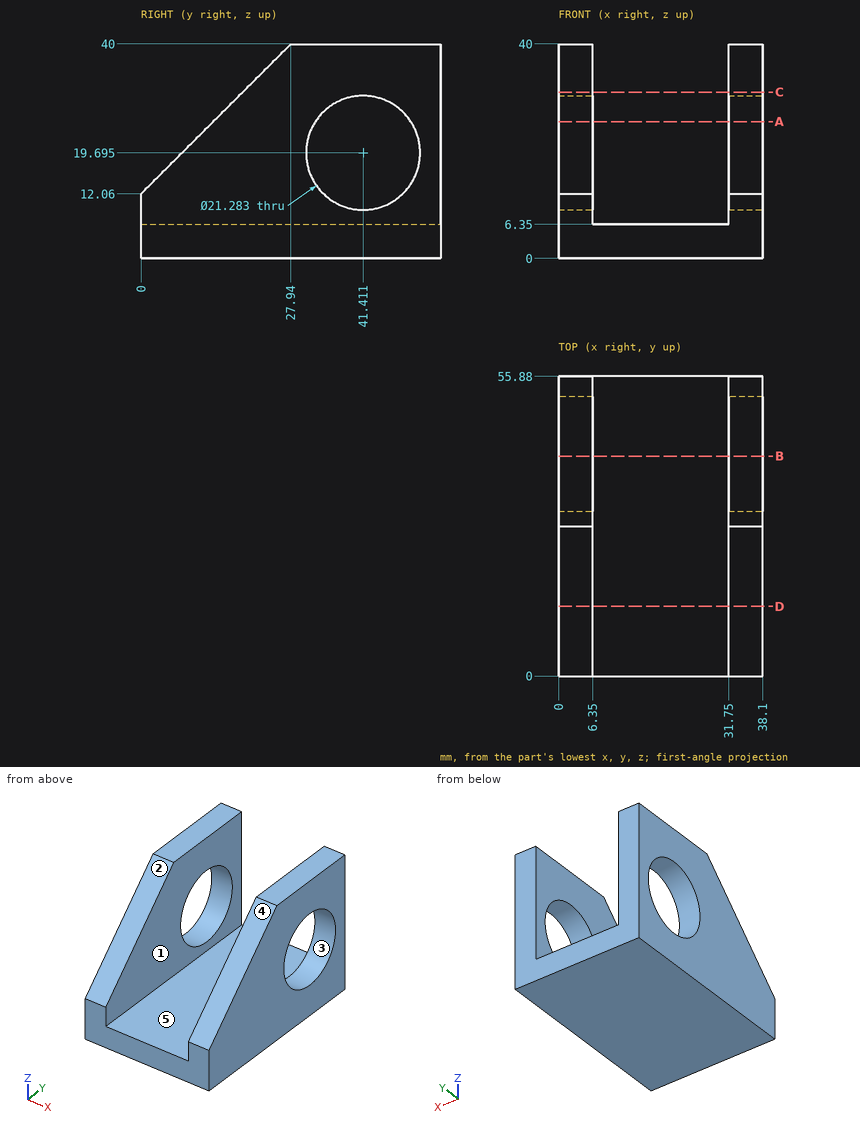
The figure shows three views and two pictorial views of one solid part (mm, origin at its lowest corner). Answer the questions. A direction names the side the tool comes from. Coordinates: 2 decimals unless noted, no trailing zeros. Loops run counter-clockwise (first coordinate to the right, second up) from the corner with the lowest first, then second, coordinate; pieces in that order, holes last. Notation, with made-up numbers: (0.25, 24) -> (19.25, 24) arc R24 ccw to (19.25, 39) -> close; hole circle Ø6 at (3.5, -12.5). An arc over 180 degrees is marked (long way). Write item = value, one per line. Start each with the question number.
1) A cutting plane is placed at C-C (z = 31). Give the vertices of the cut face in (x, y).
2) Given pin 1 Ø13 at (y, z) = (41.41, 19.7) entering from +X; pin 2 Ø3 at (x, y) = (17, 40.5) entering from +Z, each flat-ended and moving along its own axis, determine where each tip first touches the part or whether it passes through.
3) A tool of negligible diameter and unlimited length cuts with its end or side. For the marked faces 4 and 5, from which of +Z, -Z, +X, -X, +Y, -Y can it reach the whole face along a straight path? Write none if from no direction.
4) A cutting plane is placed at D-D (y = 13). Give the vertices of the cut face in (x, z).
5) Straight lines are drawn through the part: line 1 (X direction, y = 47, z = 36.5); line 2 (Z direction, x = 15, y = 22.5); line 3 (Z direction, x = 32, y = 50). For each, find the intervals that lie inside material, in ascending order. Write a range as from..to.
6) A cutting plane is placed at B-B (y = 41). Give the vertices of the cut face in (x, z), then the cut area to 3 significant figures.
7) A cutting plane is placed at A-A (z = 25.5). Give the vertices of the cut face in (x, y).
8) The mould has two halves that part along Y. Classify the marked faces 1, 2 and 3: released by +Y, released by -Y, zero draft, split by the parting line, or undercut.
Responses:
q1.outline = (0, 18.94) -> (6.35, 18.94) -> (6.35, 55.88) -> (0, 55.88) -> close; (31.75, 18.94) -> (38.1, 18.94) -> (38.1, 55.88) -> (31.75, 55.88) -> close
q2.pin_1 = through
q2.pin_2 = 6.35
q3.face_4 = +Z, +X, -X, -Y
q3.face_5 = +Z, +Y, -Y
q4.outline = (0, 0) -> (38.1, 0) -> (38.1, 25.06) -> (31.75, 25.06) -> (31.75, 6.35) -> (6.35, 6.35) -> (6.35, 25.06) -> (0, 25.06) -> close
q5.line_1 = 0..6.35, 31.75..38.1
q5.line_2 = 0..6.35
q5.line_3 = 0..13.41, 25.98..40
q6.outline = (0, 0) -> (38.1, 0) -> (38.1, 9.06) -> (31.75, 9.06) -> (31.75, 6.35) -> (6.35, 6.35) -> (6.35, 9.06) -> (0, 9.06) -> close; (0, 30.33) -> (6.35, 30.33) -> (6.35, 40) -> (0, 40) -> close; (31.75, 30.33) -> (38.1, 30.33) -> (38.1, 40) -> (31.75, 40) -> close
q6.area = 399 mm²
q7.outline = (0, 13.44) -> (6.35, 13.44) -> (6.35, 32.49) -> (0, 32.49) -> close; (0, 50.33) -> (6.35, 50.33) -> (6.35, 55.88) -> (0, 55.88) -> close; (31.75, 13.44) -> (38.1, 13.44) -> (38.1, 32.49) -> (31.75, 32.49) -> close; (31.75, 50.33) -> (38.1, 50.33) -> (38.1, 55.88) -> (31.75, 55.88) -> close
q8.face_1 = zero draft
q8.face_2 = released by -Y
q8.face_3 = undercut
